Autodesk Inventor part; units mm, degrees
ref_plane "YZ Plane" through (0, 0, 0) normal (1, 0, 0) x (0, 1, 0)
ref_plane "XZ Plane" through (0, 0, 0) normal (0, 1, 0) x (-1, 0, 0)
ref_plane "XY Plane" through (0, 0, 0) normal (0, 0, 1) x (1, 0, 0)
sketch "Esboço1" plane through (0, 0, 0) normal (0, 0, 1) x (1, 0, 0)
  circle A0 centre (0, 0) radius 14.34
  circle A1 centre (0, -0.3472) radius 100
  circle A2 centre (0, 75) radius 10
  circle A3 centre (-65.2526, -38.0208) radius 10
  circle A4 centre (65.2526, -38.0208) radius 10
  dimension "d0" = 200
  dimension "d1" = 20
  dimension "d2" = 75
  dimension "d5" = 360
extrude "Extrusão1" add sketch "Esboço1" along normal blind 25
properties part number "Disco da Valvula Inventor"
The listing builds one solid part. Answer for the finished solid, in the listing's coordinates (mm). Give positions to 0.01 mm unless a question says otherwise; leave off trailing zeros. Write each loop counter-clockwise with the first axis right and the second up, starting at its lowest first coordinate (ties: lowest second). Pieces come first, ordered by that corner, then holes.
Item 1: Section A-A, the plane x = 0 is taken. Write down the section's boundary in (y, z).
Item 2: Section B-B, the plane y = -35 is taken. Write down the section's boundary in (x, z).
Item 3: Determine the mould class of faces 1 (the flat face through (21, 1, 25)), 2 (the cylindrical face through (-21.678, 97.275, 12.325)), 3 (the cylindrical face through (-3.1, 14, 12.3)) for opening direction X: released by +X, released by -X, zero draft, split by the parting line, or undercut.
Item 4: Section C-C, the plane x = 71.5 is taken. Write down the section's boundary in (y, z), plus the area to 3 significant figures.
Item 5: Find the intervals of material crossed by line 1 along Y through (x, z) = (0, 7); line 2 along Y through (x, z) = (-2.5, 1.75); line 3 along X through (y, z) = (-6, 7.5), in increasing order.
Item 6: Section D-D, the plane y = 75 is taken. Write down the section's boundary in (x, z), plus the area to 3 significant figures.
Item 7: Flat-ended cylindrical pins translate along their axes: P1, Ø4, axis at x = 63, z = 7, coming from the +Y side; P2, Ø16, axis at x = 65.25, y = -38.02, coming from the +Z side; P3, Ø10, axis at x = 59.5, z = 7.5, coming from the +Y side; P4, Ø8, axis at y = 7, z = 11.5, coming from the +X side. Find the tip coordinate at first contact, or state that the pin passes through.
Completed:
1. outline: (-100.35, 0) - (-14.34, 0) - (-14.34, 25) - (-100.35, 25) - close; (14.34, 0) - (65, 0) - (65, 25) - (14.34, 25) - close; (85, 0) - (99.65, 0) - (99.65, 25) - (85, 25) - close
2. outline: (-93.8, 0) - (-74.79, 0) - (-74.79, 25) - (-93.8, 25) - close; (-55.72, 0) - (55.72, 0) - (55.72, 25) - (-55.72, 25) - close; (74.79, 0) - (93.8, 0) - (93.8, 25) - (74.79, 25) - close
3. face 1: zero draft
3. face 2: split by the parting line
3. face 3: undercut
4. outline: (-70.26, 0) - (-45.83, 0) - (-45.83, 25) - (-70.26, 25) - close; (-30.21, 0) - (69.57, 0) - (69.57, 25) - (-30.21, 25) - close
4. area: 3,110 mm2
5. line 1: y = -100.35 to -14.34, 14.34 to 65, 85 to 99.65
5. line 2: y = -100.32 to -14.12, 14.12 to 65.32, 84.68 to 99.62
5. line 3: x = -99.84 to -13.02, 13.02 to 99.84
6. outline: (-65.75, 0) - (-10, 0) - (-10, 25) - (-65.75, 25) - close; (10, 0) - (65.75, 0) - (65.75, 25) - (10, 25) - close
6. area: 2,790 mm2
7. P1: stops at y = 78.89
7. P2: passes through
7. P3: stops at y = 83.5
7. P4: stops at x = 99.94
